Could you check a few things on this model? Use its own coordinates, in mm. A direction names the side the tool comes from. Give positions to 0.01 mm unless a question says otherwise; leave off trailing zeros. Loops run counter-clockwise (first coordinate to the right, second up) from the corner with the lowest first, then second, coordinate; pieces in that order, holes last. Notation, with made-up numbers: (70, 73) - (103, 73) arc R14 ccw to (103, 92) - close; hole circle Ø9 at (15, 52.25). An arc over 180 degrees is marked (long way). One line per item, written item: value. Start each with the question number.
Q1. I want a section at A-A (x = 0.75). Please give me the cut outline in (y, z).
Q2. I want a section at B-B (z = 0). Please give me the cut outline in (x, y), then the cut area to 3 significant figures.
Q3. For faces 5 (the face through (11.5, 1, 0)), 6 (the face through (9.5, 1, 0)), which set-ups out of +Z, -Z, +X, -X, +Y, -Y let a thin tool reach every point of the face, with its end or its side?
Q4. If we mould it in two halves opening along Z, with no side actions, what happens to faces 1 (the face through (4, 1, 3)), 2 (the face through (5, 1, 5)), 3 (the face through (5, 1, -3)), 4 (the face through (4, 3, -4))? For each: released by +Z, released by -Z, zero draft, split by the parting line, or undercut.
Q5. If I drill on line 1 (Z direction, x = 0.75, y = 0.65); line 2 (Z direction, x = 5.25, y = 2.8); line 3 (X direction, y = 0.9, z = -1.5), over which ranges is the centre line in solid material (lowest first)? Write a range as from..to.
Q6. I want a section at D-D (y = 0.8). Please give me the cut outline in (x, z).
Q7. I want a section at C-C (y = 2.8). Please give me the cut outline in (x, z).
Q8. I'm going to push flat-ended pins straight in: P1, Ø5, axis at x = 6.5, z = 2.5, coming from the -Y side; P2, Ø1, axis at y = 2.5, z = 2.5, coming from the -X side; P3, Ø1.5, axis at x = 7.5, z = 1.5, coming from the +Y side; P4, Ø0.6, axis at y = 2, z = 1, coming from the -X side. Where does each tip first touch, or does it pass through?
Autodesk Inventor part; units mm, degrees
ref_plane "YZ Plane" through (0, 0, 0) normal (1, 0, 0) x (0, 1, 0)
ref_plane "XZ Plane" through (0, 0, 0) normal (0, 1, 0) x (-1, 0, 0)
ref_plane "XY Plane" through (0, 0, 0) normal (0, 0, 1) x (1, 0, 0)
sketch "Sketch1" plane through (0, 0, 0) normal (0, 1, 0) x (-1, 0, 0)
  line L0 (-9, -3) -> (0, -3)
  arc A0 (0, -3) -> (0, 3) centre (0, 0) ccw
  line L1 (0, 3) -> (-9, 3)
  arc A1 (-9.5, -2.5) -> (-9, -3) centre (-9, -2.5) ccw
  line L2 (-9.5, -2.5) -> (-9.5, 2.5)
  arc A2 (-9, 3) -> (-9.5, 2.5) centre (-9, 2.5) ccw
  line L3 (0, -5) -> (-9, -5)
  arc A3 (-11.5, -2.5) -> (-9, -5) centre (-9, -2.5) ccw
  line L4 (-11.5, -2.5) -> (-11.5, 2.5)
  arc A4 (-9, 5) -> (-11.5, 2.5) centre (-9, 2.5) ccw
  line L5 (-9, 5) -> (0, 5)
  arc A5 (0, -5) -> (0, 5) centre (0, 0) ccw
  dimension "d0" = 3
  dimension "d1" = 0.5
  dimension "d2" = 9.5
  dimension "d3" = 2
extrude "Extrusion1" add sketch "Sketch1" along normal blind 3
fillet "Fillet1" radius 0.5 24 edges at (10.7678, 3, 4.2678) (11.5, 3, 0) (10.7678, 3, -4.2678) (4.5, 3, -5) (-5, 3, 0) (4.5, 3, 5) (-3, 3, 0) (4.5, 3, -3) (9.3536, 3, -2.8536) (9.5, 3, 0) (9.3536, 3, 2.8536) (4.5, 3, 3) (-3, 0, 0) (4.5, 0, 3) (9.3536, 0, 2.8536) (9.5, 0, 0) (9.3536, 0, -2.8536) (4.5, 0, -3) (10.7678, 0, -4.2678) (11.5, 0, 0) (10.7678, 0, 4.2678) (4.5, 0, 5) (-5, 0, 0) (4.5, 0, -5)
properties part number "x_iddler_cap_zip_tie" material "ABS Plastic"
Worked answers:
1. outline: (0, -4.5) arc R0.5 ccw to (0.5, -5) - (2.5, -5) arc R0.5 ccw to (3, -4.5) - (3, -3.5) arc R0.5 ccw to (2.5, -3) - (0.5, -3) arc R0.5 ccw to (0, -3.5) - close; (0, 3.5) arc R0.5 ccw to (0.5, 3) - (2.5, 3) arc R0.5 ccw to (3, 3.5) - (3, 4.5) arc R0.5 ccw to (2.5, 5) - (0.5, 5) arc R0.5 ccw to (0, 4.5) - close
2. outline: (-5, 0.5) arc R0.5 ccw to (-4.5, 0) - (-3.5, 0) arc R0.5 ccw to (-3, 0.5) - (-3, 2.5) arc R0.5 ccw to (-3.5, 3) - (-4.5, 3) arc R0.5 ccw to (-5, 2.5) - close; (9.5, 0.5) arc R0.5 ccw to (10, 0) - (11, 0) arc R0.5 ccw to (11.5, 0.5) - (11.5, 2.5) arc R0.5 ccw to (11, 3) - (10, 3) arc R0.5 ccw to (9.5, 2.5) - close
2. area: 11.6 mm²
3. face 5: +Z, -Z, +X, +Y, -Y
3. face 6: +Y, -Y
4. face 1: undercut
4. face 2: released by +Z
4. face 3: undercut
4. face 4: zero draft
5. line 1: z = -5..-3, 3..5
5. line 2: z = -4.9..-3.1, 3.1..4.9
5. line 3: x = -4.77..-2.6, 9.5..11.5
6. outline: (0, -5) - (9, -5) arc R2.5 ccw to (11.5, -2.5) - (11.5, 2.5) arc R2.5 ccw to (9, 5) - (0, 5) arc R5 ccw to start; hole (0, -3) - (9, -3) arc R0.5 ccw to (9.5, -2.5) - (9.5, 2.5) arc R0.5 ccw to (9, 3) - (0, 3) arc R3 ccw to start
7. outline: (0, -4.9) - (9, -4.9) arc R2.4 ccw to (11.4, -2.5) - (11.4, 2.5) arc R2.4 ccw to (9, 4.9) - (0, 4.9) arc R4.9 ccw to start; hole (0, -3.1) - (9, -3.1) arc R0.6 ccw to (9.6, -2.5) - (9.6, 2.5) arc R0.6 ccw to (9, 3.1) - (0, 3.1) arc R3.1 ccw to start
8. P1: stops at y = 0
8. P2: stops at x = -4.58
8. P3: passes through
8. P4: stops at x = -4.95
